from build123d import *

# Parameters (mm, degrees)
SKETCH1_W           = 95
SKETCH1_H           = 23
BOSS_EXTRUDE1_DEPTH = 4.75
SKETCH2_W           = 32.5
SKETCH2_H           = 4.75
CUT_EXTRUDE1_DEPTH  = 5.75
SKETCH4_R           = 1.5
CUT_EXTRUDE2_DEPTH  = 5.75
SKETCH5_W           = 4.75
SKETCH5_H           = 5
CUT_EXTRUDE3_DEPTH  = 5.75


with BuildPart() as part:
    # Sketch1 → Boss-Extrude1 (new body)
    with BuildSketch(Plane.XY):
        with Locations((47.5, 11.5)):
            Rectangle(SKETCH1_W, SKETCH1_H)
    extrude(amount=BOSS_EXTRUDE1_DEPTH)

    # Sketch2 → Cut-Extrude1 (cut, through all)
    with BuildSketch(Plane.XY.offset(4.75)):
        with Locations((26.25, 2.375)):
            Rectangle(SKETCH2_W, SKETCH2_H)
        with Locations((68.75, 2.375)):
            Rectangle(SKETCH2_W, SKETCH2_H)
    extrude(amount=-CUT_EXTRUDE1_DEPTH, mode=Mode.SUBTRACT)

    # Sketch4 → Cut-Extrude2 (cut, through all)
    with BuildSketch(Plane.XY.offset(4.75)):
        with Locations((10, 15)):
            Circle(SKETCH4_R)
        with Locations((85, 15)):
            Circle(SKETCH4_R)
    extrude(amount=-CUT_EXTRUDE2_DEPTH, mode=Mode.SUBTRACT)

    # Sketch5 → Cut-Extrude3 (cut, through all)
    with BuildSketch(Plane.XY.offset(4.75)):
        with Locations((2.375, 20.5)):
            Rectangle(SKETCH5_W, SKETCH5_H)
        with Locations((92.625, 20.5)):
            Rectangle(SKETCH5_W, SKETCH5_H)
    extrude(amount=-CUT_EXTRUDE3_DEPTH, mode=Mode.SUBTRACT)


solid = part.part
Could you check a few things on this model? Use its own coordinates, in mm. A direction names the side the tool comes from. Round coordinates to 2 decimals unless told otherwise and drop trailing zeros. Write each loop counter-clockwise with the first axis right and the second up, starting at its lowest first coordinate (ties: lowest second). Pieces come first, ordered by that corner, then holes. Notation, with made-up numbers: (82.25, 82) -> (89.25, 82) arc R12 ccw to (89.25, 93) -> close; hole circle Ø10 at (52, -8). An arc over 180 degrees is marked (long way). Use a Markdown table: item, result.
1. Which directions (+Z, -Z, +X, -X, +Y, -Y) give clear straight access to the entire face, cutting with the end or side of a thin tool? Please do faces 5 (the face through (95, 9, 2)), 6 (the face through (85, 2, 2)), 7 (the face through (93, 18, 2)), 8 (the face through (2, 18, 2)), 9 (the face through (47, 0, 2)).
Answer key:
| item | result |
|---|---|
| face 5 | +Z, -Z, +X, +Y, -Y |
| face 6 | +Z, -Z, -Y |
| face 7 | +Z, -Z, +X, +Y |
| face 8 | +Z, -Z, -X, +Y |
| face 9 | +Z, -Z, +X, -X, -Y |
2. If we section it at C-C (y = 3): List the corners of the cut face in (x, z) for me.
Answer key:
| item | result |
|---|---|
| outline | (0, 0) -> (10, 0) -> (10, 4.75) -> (0, 4.75) -> close; (42.5, 0) -> (52.5, 0) -> (52.5, 4.75) -> (42.5, 4.75) -> close; (85, 0) -> (95, 0) -> (95, 4.75) -> (85, 4.75) -> close |
3. If we section it at B-B (y = 15): List the corners of the cut face in (x, z) for me.
Answer key:
| item | result |
|---|---|
| outline | (0, 0) -> (8.5, 0) -> (8.5, 4.75) -> (0, 4.75) -> close; (11.5, 0) -> (83.5, 0) -> (83.5, 4.75) -> (11.5, 4.75) -> close; (86.5, 0) -> (95, 0) -> (95, 4.75) -> (86.5, 4.75) -> close |
4. If we section it at D-D (x = 30): List the corners of the cut face in (y, z) for me.
Answer key:
| item | result |
|---|---|
| outline | (4.75, 0) -> (23, 0) -> (23, 4.75) -> (4.75, 4.75) -> close |
5. If we section it at A-A (z = 1.8): List the corners of the cut face in (x, y) for me.
Answer key:
| item | result |
|---|---|
| outline | (0, 0) -> (10, 0) -> (10, 4.75) -> (42.5, 4.75) -> (42.5, 0) -> (52.5, 0) -> (52.5, 4.75) -> (85, 4.75) -> (85, 0) -> (95, 0) -> (95, 18) -> (90.25, 18) -> (90.25, 23) -> (4.75, 23) -> (4.75, 18) -> (0, 18) -> close; hole circle Ø3 at (10, 15); hole circle Ø3 at (85, 15) |
6. We'd pull the mould along X, two halves only. Please class faces 1 (the face through (90, 0, 2)), 2 (the face through (0, 9, 2)), 3 (the face through (69, 4.75, 2)), 4 (the face through (90.25, 20, 2)): +X half, -X half, draft (parallel to the pull), parting line (faces both ways), or undercut.
Answer key:
| item | result |
|---|---|
| face 1 | draft |
| face 2 | -X half |
| face 3 | undercut |
| face 4 | +X half |
7. For pin 1 Ø1.4 at (x, z) = (32, 2) entering from -Y; pin 2 Ø1.4 at (y, z) = (19.5, 3) entering from -X; pin 3 Ø1.4 at (x, z) = (1.5, 1.5) entering from +Y, each with a flat end and sliding along its axis, tell me the tip position at first contact or that it passes through.
Answer key:
| item | result |
|---|---|
| pin 1 | stops at y = 4.75 |
| pin 2 | stops at x = 4.75 |
| pin 3 | stops at y = 18 |
8. Please list where these lines run through material, in increasing order: probe 1 along X at (y, z) = (4, 0.85); probe 2 along X at (y, z) = (14.75, 3.2); probe 3 along Y at (x, z) = (22, 4.35).
Answer key:
| item | result |
|---|---|
| probe 1 | x = 0 to 10, 42.5 to 52.5, 85 to 95 |
| probe 2 | x = 0 to 8.52, 11.48 to 83.52, 86.48 to 95 |
| probe 3 | y = 4.75 to 23 |
